from build123d import *

# Parameters (mm, degrees)
SKETCH_R     = 0.65
PAD_DEPTH    = 10
POCKET_DEPTH = 10.001


with BuildPart() as part:
    # Sketch → Pad (new body)
    with BuildSketch(Plane.XY):
        with BuildLine():
            ThreePointArc((-31.438047, 12.704399), (-28.406958, 7.454399), (-25.375869, 12.704399))
            Line((-25.375869, 12.704399), (-26.891414, 15.329399))
            ThreePointArc((-26.891414, 15.329399), (-28.406958, 16.204399), (-29.922503, 15.329399))
            Line((-31.438047, 12.704399), (-29.922503, 15.329399))
        make_face()
        with Locations((-28.406958, 10.954399)):
            Circle(SKETCH_R, mode=Mode.SUBTRACT)
    extrude(amount=PAD_DEPTH)

    # Sketch001 (on Face7 of Pad) → Pocket (cut, through all)
    with BuildSketch(Plane.XY.offset(10)):
        with BuildLine():
            ThreePointArc((-30.600779, 13.234717), (-30.255847, 13.179118), (-29.906958, 13.160514))
            Line((-29.906958, 13.160514), (-26.906958, 13.160514))
            ThreePointArc((-26.906958, 13.160514), (-26.55807, 13.179118), (-26.213138, 13.234717))
            Line((-25.906958, 12.704399), (-26.213138, 13.234717))
            ThreePointArc((-25.906958, 12.704399), (-26.400902, 12.82125), (-26.906958, 12.860514))
            Line((-26.906958, 12.860514), (-29.906958, 12.860514))
            ThreePointArc((-29.906958, 12.860514), (-30.413015, 12.82125), (-30.906958, 12.704399))
            Line((-30.906958, 12.704399), (-30.600779, 13.234717))
        make_face()
    extrude(amount=-POCKET_DEPTH, mode=Mode.SUBTRACT)


solid = part.part
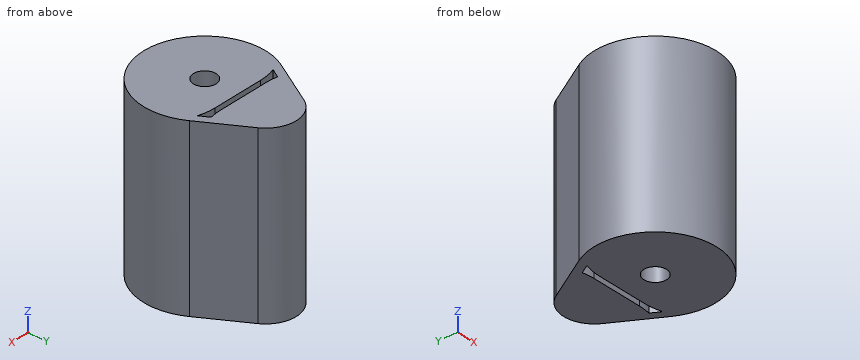
CAD build for the part. Positions are in the model's coordinates, mm. Round coordinates to 2 decimals unless told otherwise and drop trailing zeros. Write each loop counter-clockwise with the first axis right and the second up, starting at its lowest first coordinate (ties: lowest second). Pieces come first, ordered by that corner, then holes. Notation, with made-up numbers: M 2,-38 L 52,-38 A23 cw 52,-16 Z; hole C 77,51.25 d2. An arc over 180 degrees is marked long. Put each result on its own line as item: value. Start each with the question number.
1) Saw through at D-D, the plane y = 9.75. Write the cut outline in (x, z), and give its area (3 significant figures).
2) Saw through at A-A, the plane x = -28. Write the cut outline in (y, z).
3) Pin check, flat tips, straight feed: pin 1 Ø1.5 at (x, z) = (-28, 4) entering from -Y; pin 2 Ø1 at (y, z) = (15, 1.5) entering from -X; pin 3 Ø2 at (y, z) = (14.5, 8) entering from +X. Stop position of each tip, or through.
4) Drill centre lines: probe 1 along Y at (x, z) = (-28.25, 8.5); probe 2 along Y at (x, z) = (-26.75, 1); probe 3 along Y at (x, z) = (-29.5, 3.5). Where is each one in solid material? Low to high. Write a range as [from, to].
5) Saw through at B-B, the plane z = 3.25. Write the cut outline in (x, y).
6) Saw through at C-C, the plane x = -30.75. Write the cut outline in (y, z), and give its area (3 significant figures).
Resolved:
1. outline: M -31.69,0 L -25.12,0 L -25.12,10 L -31.69,10 Z
1. area: 65.7 mm²
2. outline: M 7.48,0 L 10.45,0 L 10.45,10 L 7.48,10 Z; M 11.46,0 L 12.86,0 L 12.86,10 L 11.46,10 Z; M 13.16,0 L 16.16,0 L 16.16,10 L 13.16,10 Z
3. pin 1: y = 7.45
3. pin 2: x = -30.4
3. pin 3: x = -25.84
4. probe 1: [7.46, 10.32], [11.59, 12.86], [13.16, 16.2]
4. probe 2: [7.87, 12.86], [13.16, 15.08]
4. probe 3: [7.63, 12.86], [13.16, 15.82]
5. outline: M -31.44,12.7 A3.5 ccw long -25.38,12.7 L -26.89,15.33 A1.75 ccw -29.92,15.33 Z; hole M -30.91,12.7 A3.28 cw -29.91,12.86 L -26.91,12.86 A3.28 cw -25.91,12.7 L -26.21,13.23 A3.28 cw -26.91,13.16 L -29.91,13.16 A3.28 cw -30.6,13.23 Z; hole C -28.41,10.95 d1.3
6. outline: M 8.35,0 L 12.75,0 L 12.75,10 L 8.35,10 Z; M 12.98,0 L 13.9,0 L 13.9,10 L 12.98,10 Z
6. area: 53.2 mm²
